Could you check a few things on this model? Use its own coordinates, in mm. A direction names the side the tool comes from. Give positions to 0.01 mm unless a question says otherwise; leave off trailing zeros. Order: outer loops, then holes, each group sorted by start corner. A loop starts at its lowest first (then second) coordinate and runs counter-clockwise, first axis right, second up.
from build123d import *

# Parameters (mm, degrees)
CYLINDER1886_R               = 1.5
CYLINDER1886_DEPTH           = 50
CYLINDER1888_R               = 1.5
CYLINDER1888_DEPTH           = 50
CYLINDER1887_R               = 1.5
CYLINDER1887_DEPTH           = 50
CYLINDER1885_R               = 1.5
CYLINDER1885_DEPTH           = 50
BOX794_W                     = 2
BOX794_H                     = 6
BOX794_DEPTH                 = 6
BOX797_W                     = 2
BOX797_H                     = 6
BOX797_DEPTH                 = 6
BOX795_W                     = 2
BOX795_H                     = 6
BOX795_DEPTH                 = 6
BOX796_W                     = 2
BOX796_H                     = 6
BOX796_DEPTH                 = 6
CYLINDER1871_R               = 1.5
CYLINDER1871_DEPTH           = 50
CYLINDER1871_PLACEMENT_ANGLE = 45
BOX781_W                     = 6
BOX781_H                     = 8
BOX781_DEPTH                 = 2
BOX784_W                     = 49
BOX784_H                     = 36
BOX784_DEPTH                 = 6


with BuildPart() as obj1:
    # Cylinder1886 → Cylinder1886 (new body)
    with BuildSketch(Plane(origin=(-31, 150, 72), x_dir=(1, 0, 0), z_dir=(0, -1, 0))):
        Circle(CYLINDER1886_R)
    extrude(amount=CYLINDER1886_DEPTH)


with BuildPart() as obj2:
    # Cylinder1888 → Cylinder1888 (new body)
    with BuildSketch(Plane(origin=(31, 150, 48), x_dir=(1, 0, 0), z_dir=(0, -1, 0))):
        Circle(CYLINDER1888_R)
    extrude(amount=CYLINDER1888_DEPTH)


with BuildPart() as obj3:
    # Cylinder1887 → Cylinder1887 (new body)
    with BuildSketch(Plane(origin=(31, 150, 72), x_dir=(1, 0, 0), z_dir=(0, -1, 0))):
        Circle(CYLINDER1887_R)
    extrude(amount=CYLINDER1887_DEPTH)


with BuildPart() as compound949:
    # Cylinder1885 → Cylinder1885 (new body)
    with BuildSketch(Plane(origin=(-31, 150, 48), x_dir=(1, 0, 0), z_dir=(0, -1, 0))):
        Circle(CYLINDER1885_R)
    extrude(amount=CYLINDER1885_DEPTH)

    # Compound949: union obj1, obj2, obj3
    add(obj1.part)
    add(obj2.part)
    add(obj3.part)


with BuildPart() as krychle794:
    # Box794 → Box794 (new body)
    with BuildSketch(Plane(origin=(-28, 110, 69), x_dir=(0, 1, 0), z_dir=(0, 0, 1))):
        with Locations((1, 3)):
            Rectangle(BOX794_W, BOX794_H)
    extrude(amount=BOX794_DEPTH)


with BuildPart() as krychle797:
    # Box797 → Box797 (new body)
    with BuildSketch(Plane(origin=(34, 110, 45), x_dir=(0, 1, 0), z_dir=(0, 0, 1))):
        with Locations((1, 3)):
            Rectangle(BOX797_W, BOX797_H)
    extrude(amount=BOX797_DEPTH)


with BuildPart() as krychle795:
    # Box795 → Box795 (new body)
    with BuildSketch(Plane(origin=(34, 110, 69), x_dir=(0, 1, 0), z_dir=(0, 0, 1))):
        with Locations((1, 3)):
            Rectangle(BOX795_W, BOX795_H)
    extrude(amount=BOX795_DEPTH)


with BuildPart() as compound948:
    # Box796 → Box796 (new body)
    with BuildSketch(Plane(origin=(-28, 110, 45), x_dir=(0, 1, 0), z_dir=(0, 0, 1))):
        with Locations((1, 3)):
            Rectangle(BOX796_W, BOX796_H)
    extrude(amount=BOX796_DEPTH)

    # Compound948: union Krychle794, Krychle797, Krychle795
    add(krychle794.part)
    add(krychle797.part)
    add(krychle795.part)


with BuildPart() as compound941:
    # Cylinder1871 → Cylinder1871 (new body)
    with BuildSketch(Plane.XY):
        Circle(CYLINDER1871_R)
    extrude(amount=CYLINDER1871_DEPTH)


with BuildPart() as compound941_1:
    # Cylinder1871 placement: moved
    add(compound941.part.moved(Location((-31, 101, 0))).rotate(Axis((-31, 101, 0), (0, 0, 1)), CYLINDER1871_PLACEMENT_ANGLE))


with BuildPart() as compound938:
    # Box781 → Box781 (new body)
    with BuildSketch(Plane(origin=(-27, 98, 39), x_dir=(0, 1, 0), z_dir=(0, 0, 1))):
        with Locations((3, 4)):
            Rectangle(BOX781_W, BOX781_H)
    extrude(amount=BOX781_DEPTH)


with BuildPart() as cut595:
    # Box784 → Box784 (new body)
    with BuildSketch(Plane(origin=(-34, 86, 78), x_dir=(0, 0, -1), z_dir=(1, 0, 0))):
        with Locations((24.5, 18)):
            Rectangle(BOX784_W, BOX784_H)
    extrude(amount=BOX784_DEPTH)

    # Cut586: cut Compound938
    add(compound938.part, mode=Mode.SUBTRACT)

    # Cut589: cut Compound941
    add(compound941_1.part, mode=Mode.SUBTRACT)

    # Cut594: cut Compound948
    add(compound948.part, mode=Mode.SUBTRACT)

    # Cut595: cut Compound949
    add(compound949.part, mode=Mode.SUBTRACT)


solid = cut595.part
Item 1: Imagine slicing it at B-B on z = 72. List the corners of the cut face in (x, y) for me, then the cut area to 3 significant figures.
Findings:
outline: (-34, 86) - (-28, 86) - (-28, 110) - (-29.5, 110) - (-29.5, 100) - (-32.5, 100) - (-32.5, 110) - (-34, 110) - close; (-34, 112) - (-32.5, 112) - (-32.5, 122) - (-34, 122) - close; (-29.5, 112) - (-28, 112) - (-28, 122) - (-29.5, 122) - close
area: 144 mm2
Item 2: Please list where these lines run through material, in increasing order: line 1 along Z through (x, y) = (-31, 104.5); line 2 along Z through (x, y) = (-32.9, 111.5); line 3 along X through (y, z) = (116, 72).
Findings:
line 1: z = 29 to 46.5, 49.5 to 70.5, 73.5 to 78
line 2: z = 29 to 45, 51 to 69, 75 to 78
line 3: x = -34 to -32.5, -29.5 to -28
Item 3: For pin 1 (0.9 mm diameter, centred on x = -30.5, z = 72, fed in from +Y), with a flat end and sliding along its axis, tell me the tip position at first contact or that it passes through.
Findings:
pin 1: stops at y = 100
Item 4: For faces 1 (the flat face through (-29.6, 112, 70.6)), 2 (the cylindrical face through (-29.5, 100.4, 48)), 3 (the cylindrical face through (-31.196, 99.513, 45.437)), which set-ups out of +Z, -Z, +X, -X, +Y, -Y let a thin tool reach every point of the face, with its end or its side?
Findings:
face 1: +X, -X
face 2: +Y
face 3: -Z
Item 5: Imagine slicing it at D-D on z = 35.5. List the corners of the cut face in (x, y) for me.
Findings:
outline: (-34, 86) - (-28, 86) - (-28, 122) - (-34, 122) - close; hole circle Ø3 at (-31, 101)
Item 6: We'd pull the mould along X, two halves only. Please class faces 4 (the flat face through (-31, 104, 29)), 5 (the cylindrical face through (-32.5, 100.4, 48)), 6 (the flat face through (-28, 104, 54)), 7 (the flat face through (-31, 100, 72)): +X half, -X half, draft (parallel to the pull), parting line (faces both ways), or undercut.
Findings:
face 4: draft
face 5: undercut
face 6: +X half
face 7: undercut
Item 7: Imagine slicing it at A-A on y = 110.5. List the corners of the cut face in (x, z) for me, then the cut area to 3 significant figures.
Findings:
outline: (-34, 29) - (-28, 29) - (-28, 45) - (-34, 45) - close; (-34, 51) - (-28, 51) - (-28, 69) - (-34, 69) - close; (-34, 75) - (-28, 75) - (-28, 78) - (-34, 78) - close
area: 222 mm2
Item 8: Imagine slicing it at C-C on x = -28.85. List the corners of the cut face in (y, z) for me.
Findings:
outline: (86, 29) - (122, 29) - (122, 78) - (86, 78) - close; hole (98, 39) - (104, 39) - (104, 41) - (98, 41) - close; hole (110, 45) - (112, 45) - (112, 51) - (110, 51) - close; hole (110, 69) - (112, 69) - (112, 75) - (110, 75) - close
